from build123d import *

# Parameters (mm, degrees)
BOSS_EXTRUDE1_DEPTH = 10
SKETCH2_R           = 2
CUT_EXTRUDE1_DEPTH  = 81.833161512


with BuildPart() as part:
    # Sketch1 → Boss-Extrude1 (new body)
    with BuildSketch(Plane.XY):
        with BuildLine():
            Line((52, -15.5), (52, 25.5))
            ThreePointArc((52, 25.5), (51.121320344, 27.621320344), (49, 28.5))
            Line((49, 28.5), (-49, 28.5))
            ThreePointArc((-49, 28.5), (-51.121320344, 27.621320344), (-52, 25.5))
            Line((-52, 25.5), (-52, -15.5))
            ThreePointArc((-52, -15.5), (-52.878679656, -17.621320344), (-55, -18.5))
            Line((-55, -18.5), (-65, -18.5))
            Line((-65, -18.5), (-65, -23.5))
            Line((-65, -23.5), (-52, -23.5))
            Line((-52, -23.5), (-50, -23.5))
            ThreePointArc((-50, -23.5), (-47.878679656, -22.621320344), (-47, -20.5))
            Line((-47, -20.5), (-47, 20.5))
            ThreePointArc((-47, 20.5), (-46.121320344, 22.621320344), (-44, 23.5))
            Line((-44, 23.5), (44, 23.5))
            ThreePointArc((44, 23.5), (46.121320344, 22.621320344), (47, 20.5))
            Line((47, 20.5), (47, -20.5))
            ThreePointArc((47, -20.5), (47.878679656, -22.621320344), (50, -23.5))
            Line((50, -23.5), (52, -23.5))
            Line((52, -23.5), (65, -23.5))
            Line((65, -23.5), (65, -18.5))
            Line((65, -18.5), (55, -18.5))
            ThreePointArc((55, -18.5), (52.878679656, -17.621320344), (52, -15.5))
        make_face()
    extrude(amount=BOSS_EXTRUDE1_DEPTH)

    # Sketch2 → Cut-Extrude1 (cut, through all)
    with BuildSketch(Plane(origin=(0, -18.5, 0), x_dir=(1, 0, 0), z_dir=(0, 1, 0))):
        with Locations(Location((-60, -5, 0), (0, 0, 270))):
            Circle(SKETCH2_R)
        with Locations(Location((60, -5, 0), (0, 0, 270))):
            Circle(SKETCH2_R)
    extrude(amount=-CUT_EXTRUDE1_DEPTH, mode=Mode.SUBTRACT)


solid = part.part
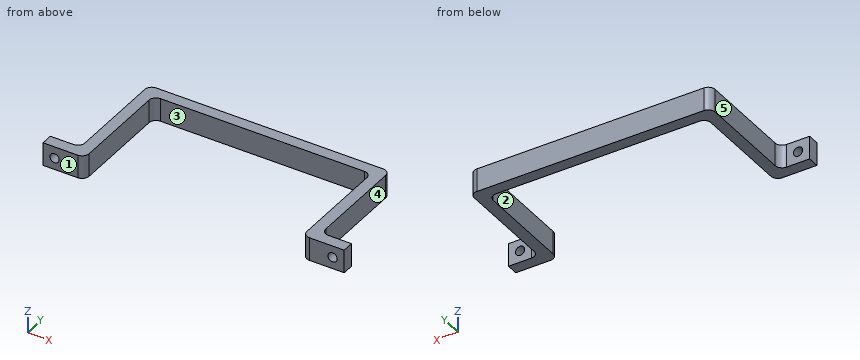
Work out the finished part from the listing and answer in its coordinate system (mm). Face numbers are marked on the shaded views. A direction names the side the tool comes from. Round coordinates to 2 decimals unless told otherwise and drop trailing zeros. Write each loop counter-clockwise with the first axis right and the second up, starting at its lowest first coordinate (ties: lowest second). Pieces come first, ordered by that corner, then holes. Notation, with made-up numbers: (-39, 12) - (-18, 12) arc R28 ccw to (-18, 37) - close; hole circle Ø1 at (77, 39). An arc over 180 degrees is marked (long way). Answer in a Markdown table with one row per item. Add a question column.
1. Given pin 1 (4 mm diameter, centred on x = -34, z = 5.5, fed in from -Y); pin 2 (5 mm diameter, centred on y = 3, z = 5.5, fed in from -X); pin 3 (3 mm diameter, centred on x = 61.5, z = 5.5, fed in from +Y), each flat-ended and moving along its own axis, determine where each tip first touches the part or whether it passes through.
2. A cutting plane is placed at B-B, the plane x = 60. Determine the outline of the cut face in (y, z).
3. A cutting plane is placed at A-A, the plane y = 10. Determine the outline of the cut face in (x, z).
4. For the marked faces 1 and 2, determine the directions among +Z, -Z, +X, -X, +Y, -Y from which every point of the face is accessible in a straight line to the end or side of a thin tool.
5. A cutting plane is placed at C-C, the plane z = 5. Determine the outline of the cut face in (x, y), and give its area (3 significant figures).
6. The mould has two halves that part along X. Classify the marked faces 3, 4 and 5: +X half, -X half, draft (parallel to the pull), parting line (faces both ways), or undercut.
7. Find the intervals of material crossed by line 1 along X through (y, z) = (-5, 3); line 2 along X through (y, z) = (-20, 5); line 3 along Y through (x, z) = (38.5, 6.25), in increasing order. Write a range as from..to.
8. A cutting plane is placed at D-D, the plane x = 39. Determine the outline of the cut face in (y, z).
Worked out:
| question | item | result |
|---|---|---|
| 1 | pin 1 | y = 23.5 |
| 1 | pin 2 | x = -52 |
| 1 | pin 3 | y = -18.5 |
| 2 | outline | (-23.5, 0) - (-18.5, 0) - (-18.5, 3) - (-23.5, 3) - close; (-23.5, 7) - (-18.5, 7) - (-18.5, 10) - (-23.5, 10) - close |
| 3 | outline | (-52, 0) - (-47, 0) - (-47, 10) - (-52, 10) - close; (47, 0) - (52, 0) - (52, 10) - (47, 10) - close |
| 4 | face 1 | +Z, -Z, +X, -X, -Y |
| 4 | face 2 | +Z, -Z, -Y |
| 5 | outline | (-65, -23.5) - (-62, -23.5) - (-62, -18.5) - (-65, -18.5) - close; (-58, -23.5) - (-50, -23.5) arc R3 ccw to (-47, -20.5) - (-47, 20.5) arc R3 cw to (-44, 23.5) - (44, 23.5) arc R3 cw to (47, 20.5) - (47, -20.5) arc R3 ccw to (50, -23.5) - (58, -23.5) - (58, -18.5) - (55, -18.5) arc R3 cw to (52, -15.5) - (52, 25.5) arc R3 ccw to (49, 28.5) - (-49, 28.5) arc R3 ccw to (-52, 25.5) - (-52, -15.5) arc R3 cw to (-55, -18.5) - (-58, -18.5) - close; (62, -23.5) - (65, -23.5) - (65, -18.5) - (62, -18.5) - close |
| 5 | area | 1,080 mm^2 |
| 6 | face 3 | undercut |
| 6 | face 4 | +X half |
| 6 | face 5 | -X half |
| 7 | line 1 | -52..-47, 47..52 |
| 7 | line 2 | -65..-62, -58..-47, 47..58, 62..65 |
| 7 | line 3 | 23.5..28.5 |
| 8 | outline | (23.5, 0) - (28.5, 0) - (28.5, 10) - (23.5, 10) - close |
